Geometry: final body of the model. Coordinates: model frame, mm. Face numbers are marked on the shaded views. A direction names the side the tool comes from. Give positions to 0.01 mm unless a question says otherwise; leave off trailing zeros. Order: outer loops, then holes, each group sorted by start corner. A loop starts at its lowest first (then second) coordinate and runs counter-clockwise, first axis right, second up. Notation, with made-up numbers: M 3,-10.5 L 44,-10.5 A12 ccw 44,7.5 Z; hole C 54.5,49 d8. An arc over 180 degrees is marked long. Write item = value, one per line. Start each with the question number.
from build123d import *

# Parameters (mm, degrees)
SM_BASE_FLANGE_1_DEPTH = 17
SKETCH_6_R             = 11.5
CUT_EXTRUDE_1_DEPTH    = 43.95346319
FILLET_1_R             = 1


# Sheet-metal steps are written as plain solids
with BuildPart() as part:
    # Sketch 1 → Базовая кромка1 (new, symmetric)
    with BuildSketch(Plane(origin=(0, 0, 0), x_dir=(0, 0, -1), z_dir=(1, 0, 0))):
        with BuildLine():
            Line((-34, 0), (-1.6, 0))
            ThreePointArc((-1.6, 0), (-0.46862915, 0.46862915), (0, 1.6))
            Line((0, 1.6), (0, 20))
            Line((0, 20), (1.5, 20))
            Line((1.5, 20), (1.5, 1.6))
            ThreePointArc((1.5, 1.6), (0.592031022, -0.592031022), (-1.6, -1.5))
            Line((-1.6, -1.5), (-34, -1.5))
            Line((-34, -1.5), (-34, 0))
        make_face()
    extrude(amount=SM_BASE_FLANGE_1_DEPTH, both=True)

    # Эскиз6 → Вырез-Вытянуть1 (cut, through all)
    with BuildSketch(Plane(origin=(0, 0, 0), x_dir=(1, 0, 0), z_dir=(0, 1, 0))):
        with Locations(Location((0, -18, 0), (0, 0, 270))):
            Circle(SKETCH_6_R)
    extrude(amount=-CUT_EXTRUDE_1_DEPTH, mode=Mode.SUBTRACT)

    # Скругление1
    fillet_1_edges = [part.edges().sort_by_distance(p)[0] for p in [
        (17, -0.75, 34),
        (17, 20, -0.75),
        (-17, -0.75, 34),
        (-17, 20, -0.75),
    ]]
    fillet(fillet_1_edges, radius=FILLET_1_R)


solid = part.part
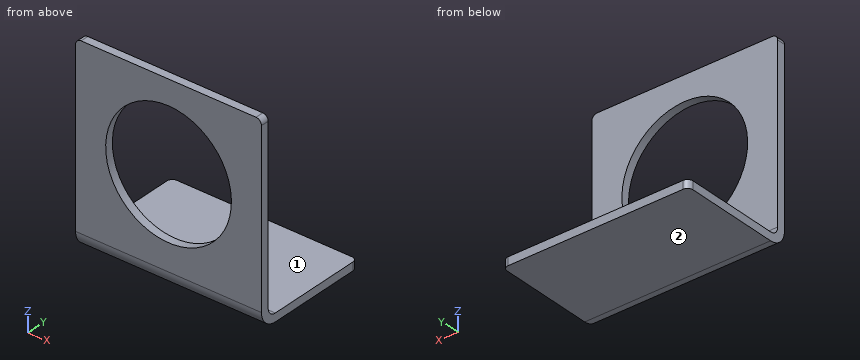
1) Cut plane C-C (x = 14.5). Return loops of the section in (y, z), plus the area to 3 significant figures.
2) Cut plane A-A (x = 0). Return loops of the section in (y, z), plus the area to 3 significant figures.
3) Access query for the marked faces 1 and 2. Directions: +Z, -Z, +X, -X, +Y, -Y. A direction counts if a zero-diameter tool reaches every point of the face in a straight line with its end or side. Return the directions, or none.
4) Cut plane D-D (z = 9.5). Return loops of the section in (x, y), plus the area to 3 significant figures.
5) Ray query, L1, parallel to X at y = -0.75, z = 18; L2, parallel to Z at x = -6.5, y = 15. Return the intervals inside material, ascending.
6) Cut plane B-B (z = 18). Return loops of the section in (x, y).
7) Pin query (flat end, axial travel): pin 1 Ø10 at (y, z) = (8.5, 16) entering from -X; pin 2 Ø12 at (x, z) = (7.5, 10) entering from +Y. Return the tip coordinate at first contact, or that it passes through.
Reply:
q1.outline = M -1.5,1.6 A3.1 ccw 1.6,-1.5 L 20,-1.5 L 20,0 L 1.6,0 A1.6 cw 0,1.6 L 0,34 L -1.5,34 Z
q1.area = 81.7 mm²
q2.outline = M -1.5,1.6 A3.1 ccw 1.6,-1.5 L 20,-1.5 L 20,0 L 1.6,0 A1.6 cw 0,1.6 L 0,6.5 L -1.5,6.5 Z; M -1.5,29.5 L 0,29.5 L 0,34 L -1.5,34 Z
q2.area = 47.2 mm²
q3.face_1 = +Z, +X, -X, +Y
q3.face_2 = -Z, +X, -X, +Y, -Y
q4.outline = M -17,-1.5 L -7.75,-1.5 L -7.75,0 L -17,0 Z; M 7.75,-1.5 L 17,-1.5 L 17,0 L 7.75,0 Z
q4.area = 27.8 mm²
q5.L1 = -17 to -11.5, 11.5 to 17
q5.L2 = -1.5 to 0
q6.outline = M -17,-1.5 L -11.5,-1.5 L -11.5,0 L -17,0 Z; M 11.5,-1.5 L 17,-1.5 L 17,0 L 11.5,0 Z
q7.pin_1 = through
q7.pin_2 = 0
